Build history of the part. All positions in model axes, mm. Round coordinates to 2 decimals unless told otherwise and drop trailing zeros. Write each loop counter-clockwise with the first axis right and the second up, starting at its lowest first coordinate (ties: lowest second). Pieces come first, ordered by that corner, then holes. Notation, with made-up numbers: M 6.5,85 L 40.5,85 A34 ccw 40.5,124 Z; hole C 60,13 d11. An arc over 180 degrees is marked long. Use a Markdown table: item, result.
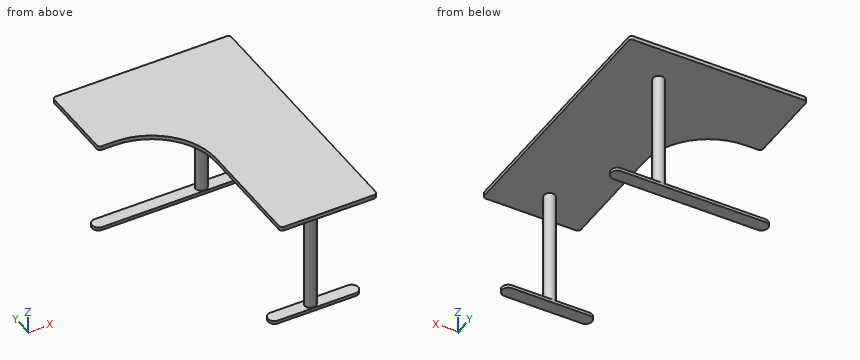
from build123d import *

# Parameters (mm, degrees)
F1_DEPTH = 2.5
F2_R     = 3.5
F3_DEPTH = 75
F5_DEPTH = 2


with BuildPart() as f1:
    # F0 (on Top) → F1 (new body)
    with BuildSketch(Plane.XY):
        with BuildLine():
            ThreePointArc((0, -2), (-0.585786, -0.585786), (-2, 0))
            Line((-2, 0), (-108, 0))
            ThreePointArc((-108, 0), (-109.414214, -0.585786), (-110, -2))
            Line((-110, -2), (-110, -158))
            ThreePointArc((-110, -158), (-109.414214, -159.414214), (-108, -160))
            Line((-108, -160), (-52, -160))
            ThreePointArc((-52, -160), (-50.585786, -159.414214), (-50, -158))
            Line((-50, -158), (-50, -90))
            ThreePointArc((-50, -90), (-38.284271, -61.715729), (-10, -50))
            Line((-10, -50), (-2, -50))
            ThreePointArc((-2, -50), (-0.585786, -49.414214), (0, -48))
            Line((0, -48), (0, -2))
        make_face()
    extrude(amount=F1_DEPTH)

    # F2 (on face) → F3 (join)
    with BuildSketch(Plane(origin=(0, 0, 0), x_dir=(1, 0, 0), z_dir=(0, 0, -1))):
        with Locations((-78.837842, 141.606882)):
            Circle(F2_R)
        with Locations((-78.837842, 23.552824)):
            Circle(F2_R)
    extrude(amount=F3_DEPTH)

    # F4 (on face) → F5 (join)
    with BuildSketch(Plane(origin=(0, 0, -75), x_dir=(1, 0, 0), z_dir=(0, 0, -1))):
        with BuildLine():
            ThreePointArc((-56.533181, 137.606882), (-52.533181, 141.606882), (-56.533181, 145.606882))
            Line((-56.533181, 145.606882), (-104.533181, 145.606882))
            ThreePointArc((-104.533181, 145.606882), (-108.533181, 141.606882), (-104.533181, 137.606882))
            Line((-104.533181, 137.606882), (-56.533181, 137.606882))
        make_face()
        with BuildLine():
            ThreePointArc((-82.337842, 141.606882), (-78.837842, 145.106882), (-75.337842, 141.606882))
            ThreePointArc((-75.337842, 141.606882), (-78.837842, 138.106882), (-82.337842, 141.606882))
        make_face(mode=Mode.SUBTRACT)
        with BuildLine():
            ThreePointArc((-104.533181, 27.552824), (-108.533181, 23.552824), (-104.533181, 19.552824))
            Line((-104.533181, 19.552824), (-15.066023, 19.552824))
            ThreePointArc((-15.066023, 19.552824), (-11.066023, 23.552824), (-15.066023, 27.552824))
            Line((-15.066023, 27.552824), (-104.533181, 27.552824))
        make_face()
        with BuildLine():
            ThreePointArc((-82.337842, 23.552824), (-78.837842, 27.052824), (-75.337842, 23.552824))
            ThreePointArc((-75.337842, 23.552824), (-78.837842, 20.052824), (-82.337842, 23.552824))
        make_face(mode=Mode.SUBTRACT)
        with BuildLine():
            ThreePointArc((-82.337842, 23.552824), (-78.837842, 20.052824), (-75.337842, 23.552824))
            Line((-75.337842, 23.552824), (-82.337842, 23.552824))
        make_face()
    extrude(amount=-F5_DEPTH)


with BuildPart() as f6_1:
    # F6: instance of F1
    add(f1.part.mirror(Plane.YZ))


solid = f6_1.part
Q1. Cut at A-A on x = 45. Give the cut face in (y, z).
Response values:
| item | result |
|---|---|
| outline | M -70.64,0 L 0,0 L 0,2.5 L -70.64,2.5 Z; M -27.55,-75 L -19.55,-75 L -19.55,-73 L -27.55,-73 Z |
Q2. Drill centre lines: L1, parallel to Z at x = 47, y = -24; L2, parallel to Z at x = 34, y = -29; L3, parallel to Y at x = 82, z = -54. Where is each one in solid material? Low to high.
Response values:
| item | result |
|---|---|
| L1 | z = -75 to -73, 0 to 2.5 |
| L2 | z = 0 to 2.5 |
| L3 | y = -143.11 to -140.11, -25.05 to -22.05 |
Q3. Cut at B-B on y = -16. Give the cut face in (x, z), and give its area (3 significant figures).
Response values:
| item | result |
|---|---|
| outline | M 0,0 L 110,0 L 110,2.5 L 0,2.5 Z |
| area | 275 mm2 |
Q4. Cut at D-D on x = 21. Give the cut face in (y, z), and give its area (3 significant figures).
Response values:
| item | result |
|---|---|
| outline | M -51.54,0 L 0,0 L 0,2.5 L -51.54,2.5 Z; M -27.55,-75 L -19.55,-75 L -19.55,-73 L -27.55,-73 Z |
| area | 145 mm2 |
Q5. Drop flat-ended pins along their axis: P1, Ø1, axis at x = 71, z = -73.5, coming from the -Y side; P2, Ø0.6, axis at x = 89.5, z = -74, coming from the +Y side; P3, Ø3, axis at y = -126.5, z = 2, coming from the -X side. Give the stop position or say it passes through.
Response values:
| item | result |
|---|---|
| P1 | stops at y = -145.61 |
| P2 | stops at y = -19.55 |
| P3 | stops at x = 50 |
Q6. Cut at C-C on z = -42. Give the cut face in (x, y).
Response values:
| item | result |
|---|---|
| outline | C 78.84,-141.61 d7; C 78.84,-23.55 d7 |
